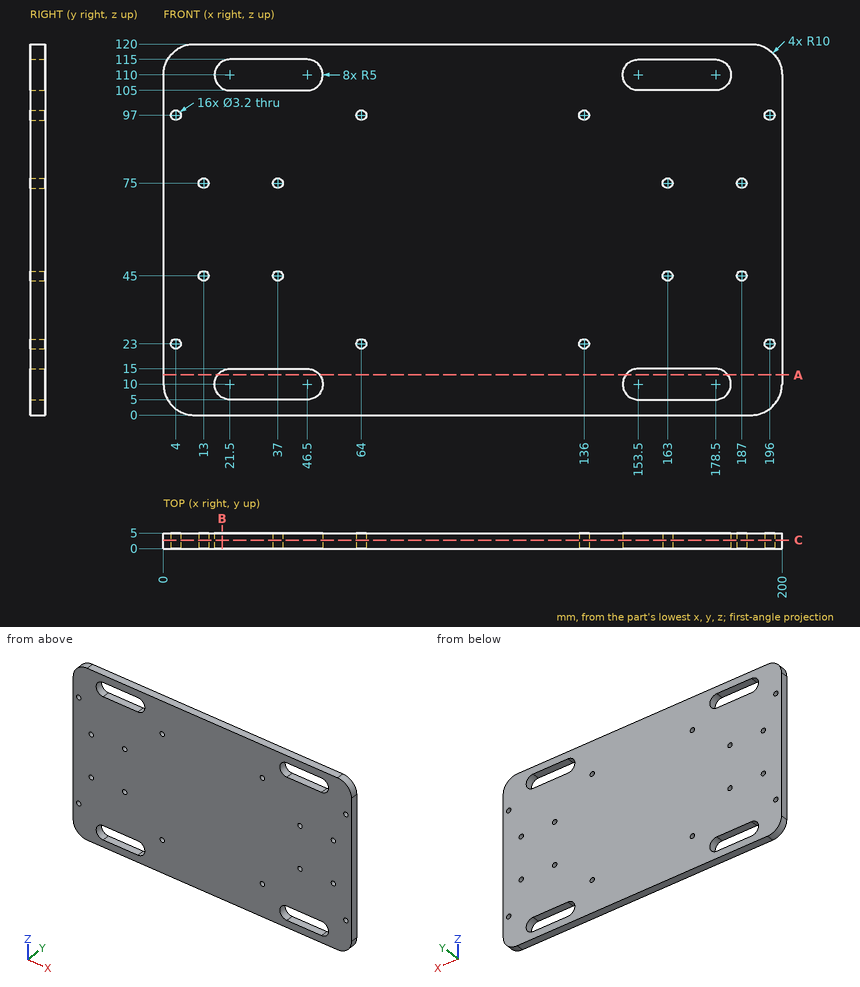
Job drawing, mm, ordinate dimensions from the low corner. One solid piece. Coordinates: 2 decimals unless noted, no trailing zeros. Loops run counter-clockwise (first coordinate to the right, second up) from the corner with the lowest first, then second, coordinate; pieces in that order, holes last. Notation, with made-up numbers: (-32, -31.5) - (20, -31.5) arc R20 cw to (20, -13.5) - close; hole circle Ø2 at (87, 52.5). An arc over 180 degrees is marked (long way). Answer as a JSON object with one key per item and string values. Group by question number.
(1) Probe line 1 along X through (y, z) = (2.2, 45); line 2 along X through (y, z) = (3.9, 23); line 3 along X through (y, z) = (4.1, 110). List the from-to ranges inside material, lowest first.
(2) Flat gauge pin, fed straight in: pin 1 (1.9 mm diameter, centred on x = 187, z = 75, fed in from -Y). Where does the tip first touch, or does it go through?
(3) Cut at C-C (y = 2.7). State how many separate pieces and enclosed holes the cut face has, then the cut area to 3 significant figures.
(4) Cut at B-B (x = 19). Give the cut face in (y, z), then the cut area to 3 significant figures.
(5) Cut at A-A (z = 13). Give the cut face in (x, y).
Geometry says:
{
 "1": {"line 1": "x = 0 to 11.4, 14.6 to 35.4, 38.6 to 161.4, 164.6 to 185.4, 188.6 to 200", "line 2": "x = 0 to 2.4, 5.6 to 62.4, 65.6 to 134.4, 137.6 to 194.4, 197.6 to 200", "line 3": "x = 0 to 16.5, 51.5 to 148.5, 183.5 to 200"},
 "2": {"pin 1": "passes through"},
 "3": {"separate pieces": "1", "enclosed holes": "20", "area": "22,500 mm^2"},
 "4": {"outline": "(0, 0) - (5, 0) - (5, 5.67) - (0, 5.67) - close; (0, 14.33) - (5, 14.33) - (5, 105.67) - (0, 105.67) - close; (0, 114.33) - (5, 114.33) - (5, 120) - (0, 120) - close", "area": "513 mm^2"},
 "5": {"outline": "(0, 0) - (17.5, 0) - (17.5, 5) - (0, 5) - close; (50.5, 0) - (149.5, 0) - (149.5, 5) - (50.5, 5) - close; (182.5, 0) - (200, 0) - (200, 5) - (182.5, 5) - close"}
}
